Design review of the part built by this model. Coordinates are the model's own, in mm. A direction names the side the tool comes from. Coordinates: 2 decimals unless noted, no trailing zeros. Write each loop counter-clockwise with the first axis right and the second up, starting at its lowest first coordinate (ties: lowest second). Pieces come first, ordered by that corner, then holes. Notation, with made-up numbers: (72, 6) - (79, 6) arc R20 ccw to (79, 38) - close; hole circle Ø3 at (-27.5, 30). An arc over 180 degrees is marked (long way). Answer as a JSON object with one key per item and string values.
Autodesk Inventor part; units mm, degrees
ref_plane "bolt2_to_body_XY" through (-10, 35.5, 0) normal (0, 1, 0) x (1, 0, 0)
ref_plane "bolt2_to_body_YZ" through (-10, 35.5, 0) normal (1, 0, 0) x (0, 0, -1)
ref_plane "bolt2_to_body_ZX" through (-10, 35.5, 0) normal (0, 0, -1) x (0, 1, 0)
sketch "Sketch_10" plane through (0, 0, 0) normal (0, 0, 1) x (1, 0, 0)
  line L0 (-16, 29) -> (-16, 0)
  line L1 (-16, 0) -> (16, 0)
  line L2 (16, 0) -> (16, 29)
  line L3 (16, 29) -> (4.899, 29)
  arc A0 (-4.899, 29) -> (4.899, 29) centre (0, 30) ccw
  line L4 (-4.899, 29) -> (-16, 29)
extrude "Extrusion1" add sketch "Sketch_10" along normal mid plane 12
sketch "Sketch2" plane through (4.899, 29, 6) normal (0, 1, 0) x (1, 0, 0)
  point P0 (5.101, 6)
hole "Hole1" at (10, 29, 0) direction (0, -1, 0) diameter 3.242 depth 6.0641 tip angle 120 countersink diameter 4 countersink angle 90
sketch "Sketch3" plane through (-16, 29, 6) normal (0, 1, 0) x (1, 0, 0)
  point P0 (6, 6)
hole "Hole2" at (-10, 29, 0) direction (0, -1, 0) diameter 3.242 depth 6.0641 tip angle 120 countersink diameter 4 countersink angle 90
sketch "Sketch_2" plane through (0, 0, 0) normal (0, 0, 1) x (1, 0, 0)
  circle A0 centre (10, 5) radius 2.25
extrude "Extrusion2" cut sketch "Sketch_2" along normal mid plane 12
sketch "Sketch_3" plane through (0, 0, 0) normal (0, 0, 1) x (1, 0, 0)
  circle A0 centre (-10, 5) radius 2.25
extrude "Extrusion3" cut sketch "Sketch_3" along normal mid plane 12
ref_plane "bolt2_to_body_XY" through (-10, 35.5, 0) normal (0, 1, 0) x (1, 0, 0)
ref_plane "bolt2_to_body_YZ" through (-10, 35.5, 0) normal (1, 0, 0) x (0, 0, -1)
ref_plane "bolt2_to_body_ZX" through (-10, 35.5, 0) normal (0, 0, -1) x (0, 1, 0)
ref_plane "bolt_to_body_XY" through (10, 35.5, 0) normal (0, 1, 0) x (1, 0, 0)
ref_plane "bolt_to_body_YZ" through (10, 35.5, 0) normal (1, 0, 0) x (0, 0, -1)
ref_plane "bolt_to_body_ZX" through (10, 35.5, 0) normal (0, 0, -1) x (0, 1, 0)
ref_plane "p_to_body_XY" through (0, 0, 0) normal (0, 1, 0) x (1, 0, 0)
ref_plane "p_to_body_YZ" through (0, 0, 0) normal (1, 0, 0) x (0, 0, -1)
ref_plane "p_to_body_ZX" through (0, 0, 0) normal (0, 0, -1) x (0, 1, 0)
properties part number "SHZA10-30_b"
(1) Tool access review of faces 5 (the face through (8.393, 25.739, -0.211)), 6 (the face through (-16, 15, 0)): name each direction out of +Z, -Z, +X, -X, +Y, -Y from which nothing blocks a thin tool from reaching the whole face with its end or side.
Solved:
{"face 5": "+Y", "face 6": "+Z, -Z, -X, +Y, -Y"}
(2) To check wall thickness, follow line 1 (Z direction, x = -10, y = 24.65); line 2 (Y direction, x = 10, z = 2); line 3 (X direction, y = 6.75, z = 4). State the ranges of each line that lie inside material, in increasing order. Write a range as from..to.
Solved:
{"line 1": "z = -6..-1.62, 1.62..6", "line 2": "y = 0..2.75, 7.25..29", "line 3": "x = -16..-11.41, -8.59..8.59, 11.41..16"}
(3) For pin 1 (4 mm diameter, centred on x = -10, y = 5, fed in from -Z); pin 2 (1 mm diameter, centred on x = 11, z = 0, fed in from +Y), all flat-tipped, find the tip position at first contact; note any pin that passes through.
Solved:
{"pin 1": "passes through", "pin 2": "stops at y = 22.87"}
(4) The part is to be moulded in two halves that separate along Z. For faces 1 (the face through (-10, 22, 0)), 2 (the face through (12, 29, -1)), 3 (the face through (10, 22, 0)), 4 (the face through (0, 15, 6)), say which applies: pulls with the +Z half, pulls with the -Z half, needs draft (parallel to the pull), parting line crosses it, or undercut.
Solved:
{"face 1": "undercut", "face 2": "needs draft", "face 3": "undercut", "face 4": "pulls with the +Z half"}
(5) Take a section at D-D, the plane x = -3. Write out the cut boundary in (y, z), and give its area (3 significant figures).
Solved:
{"outline": "(0, -6) - (26, -6) - (26, 6) - (0, 6) - close", "area": "312 mm^2"}
(6) Take a section at A-A, the plane z = -4.75. Write out the cut boundary in (x, y), and give its area (3 significant figures).
Solved:
{"outline": "(-16, 0) - (16, 0) - (16, 29) - (4.9, 29) arc R5 cw to (-4.9, 29) - (-16, 29) - close; hole circle Ø4.5 at (-10, 5); hole circle Ø4.5 at (10, 5)", "area": "867 mm^2"}
(7) Take a section at C-C, the plane y = 5. Write out the cut boundary in (x, z), and give its area (3 significant figures).
Solved:
{"outline": "(-16, -6) - (-12.25, -6) - (-12.25, 6) - (-16, 6) - close; (-7.75, -6) - (7.75, -6) - (7.75, 6) - (-7.75, 6) - close; (12.25, -6) - (16, -6) - (16, 6) - (12.25, 6) - close", "area": "276 mm^2"}
(8) Take a section at B-B, the plane y = 26.25. Write out the cut boundary in (x, z), and give its area (3 significant figures).
Solved:
{"outline": "(-16, -6) - (-3.31, -6) - (-3.31, 6) - (-16, 6) - close; (3.31, -6) - (16, -6) - (16, 6) - (3.31, 6) - close; hole circle Ø3.24 at (-10, 0); hole circle Ø3.24 at (10, 0)", "area": "288 mm^2"}
